Source: CAD feature listing. Evaluate the final solid. Frame: model axes, mm. A direction names the side the tool comes from. Give positions to 0.01 mm unless a question says otherwise; leave off trailing zeros. Write each loop counter-clockwise with the first axis right and the second up, starting at its lowest first coordinate (ties: lowest second). Pieces come first, ordered by that corner, then holes. Notation, with made-up numbers: (40, -19) -> (65, -19) arc R34 ccw to (65, 14) -> close; hole circle Ø2 at (-13, 7). An arc over 180 degrees is marked (long way). Answer as a JSON object with one key per item and string values. Group by question number.
Item 1: Section query C-C on x = -83.5. Return the cut outline in (y, z), plus the area to 3 significant figures.
Item 2: Section query B-B on y = 29.5. Return the cut outline in (x, z).
Item 3: First-contact query: pin 1 Ø1.5 at (x, y) = (-53.5, 19) entering from +Z. Flat tip, straight axial feed; report the tip coordinate or a pass-through.
Item 4: Ray query, probe 1 along X at (y, z) = (51, 39); probe 2 along Y at (x, z) = (-96, 23.5); probe 3 along Z at (x, y) = (-35, 24). Return the intervals inside material, ascending. Write a range as from..to.
Item 5: Section query A-A on z = 33.5. Return the cut outline in (x, y).
Item 6: Access query for faces 5 (the face through (-27, -24.393, 25)), 6 (the face through (-27, 16, 2.54)). Directions: +Z, -Z, +X, -X, +Y, -Y. A direction counts if a zero-diameter tool reaches every point of the face in a straight line with its end or side. Return the directions, or none.
Item 7: Pull-direction query (X, two-part tool) for faces 1 (the face through (-27, 55.716, 25)), 2 (the face through (48.397, 15, 26)), 3 (the face through (-100.377, 15, 26)), 4 (the face through (-102.917, 15, 25)); classes: pulls with the +X half, pulls with the -X half, needs draft (parallel to the pull), parting line crosses it, or undercut.
from build123d import *

# Parameters (mm, degrees)
F0_W     = 153.853889
F0_H     = 80.108998
F1_DEPTH = 50.8
F2_W     = 126.011554
F2_H     = 47.126646
F3_DEPTH = 25.4
F4_DEPTH = 25.4
F5_T     = -2.54


with BuildPart() as f1:
    # F0 (on Top) → F1 (new body)
    with BuildSketch(Plane.XY):
        with Locations((-25.98972, 15.661658)):
            Rectangle(F0_W, F0_H)
    extrude(amount=F1_DEPTH)

    # F2 (on face) → F3 (join)
    with BuildSketch(Plane.XY.offset(50.8)):
        with Locations((-26.755249, 16.175097)):
            Rectangle(F2_W, F2_H)
    extrude(amount=-F3_DEPTH)

    # F2 (on face) → F4 (join)
    with BuildSketch(Plane.XY.offset(50.8)):
        with Locations((-26.755249, 16.175097)):
            Rectangle(F2_W, F2_H)
    extrude(amount=-F4_DEPTH)

    # F5
    f5_openings = [f1.faces().sort_by_distance(p)[0] for p in [
        (-25.989721, 15.661658, 50.8),
    ]]
    offset(amount=F5_T, openings=f5_openings)


solid = f1.part
Worked answers:
{
 "1": {"outline": "(-24.39, 0) -> (55.72, 0) -> (55.72, 50.8) -> (53.18, 50.8) -> (53.18, 2.54) -> (-21.85, 2.54) -> (-21.85, 50.8) -> (-24.39, 50.8) -> close", "area": "449 mm^2"},
 "2": {"outline": "(-102.92, 0) -> (50.94, 0) -> (50.94, 50.8) -> (48.4, 50.8) -> (48.4, 2.54) -> (-100.38, 2.54) -> (-100.38, 50.8) -> (-102.92, 50.8) -> close"},
 "3": {"pin 1": "z = 2.54"},
 "4": {"probe 1": "-102.92..-100.38, 48.4..50.94", "probe 2": "-24.39..-21.85, 53.18..55.72", "probe 3": "0..2.54"},
 "5": {"outline": "(-102.92, -24.39) -> (50.94, -24.39) -> (50.94, 55.72) -> (-102.92, 55.72) -> close; hole (-100.38, -21.85) -> (48.4, -21.85) -> (48.4, 53.18) -> (-100.38, 53.18) -> close"},
 "6": {"face 5": "+Z, -Z, +X, -X, -Y", "face 6": "+Z"},
 "7": {"face 1": "needs draft", "face 2": "undercut", "face 3": "undercut", "face 4": "pulls with the -X half"}
}
